Geometry: final body of the model. Coordinates: model frame, mm. A direction names the side the tool comes from. Give positions to 0.01 mm unless a question says otherwise; leave off trailing zeros. Write each loop counter-clockwise with the first axis right and the second up, starting at its lowest first coordinate (ties: lowest second). Pieces come first, ordered by that corner, then holes.
Q1. Section A-A (x = 8.5). Return the cut outline in (y, z).
Q2. Section C-C (y = -94). Return the cut outline in (x, z).
Q3. Mould query, pull axis Y, two halves, no side actions, for faces 3 (the cylindrical face through (8, -89, 22)), 4 (the cylindrical face through (8.28, -82.51, 21.93)), 5 (the flat face through (8, -97.201, 9)), 6 (the flat face through (17, -98, 16)). Classes: +Y half, -Y half, draft (parallel to the pull), parting line (faces both ways), or undercut.
Q4. Section D-D (z = 12). Return the cut outline in (x, y).
Q5. Section B-B (x = 5.5). Return the cut outline in (y, z), plus the area to 3 significant figures.
Q6. Pin query (flat end, axial travel): pin 1 Ø5 at (x, z) = (7.5, 10.5) entering from +Y; pin 2 Ø5 at (x, y) = (7, -83) entering from -Z; pin 3 Ø12 at (y, z) = (-76.5, 18) entering from +X. Return the tip coordinate at first contact, or that it passes through.
Q7. Line query: line 1 (Y direction, x = 8.5, z = 22.15); line 2 (Z direction, x = 8.5, y = -97.6); line 3 (Z direction, x = 5.5, y = -82.5). Output: solid intervals per line, ascending.
Q8. Reachability of faces 1 (the flat face through (8, -86, 22.423)), 2 (the flat face through (8, -85, 21.423)) from +Z, -Z, +X, -X, +Y, -Y: full face, straight path, thin tool, end or side. Return the list, or none.
from build123d import *

# Parameters (mm, degrees)
F1_DEPTH = 17
F2_R     = 1
F3_DEPTH = 1
F4_R     = 1
F5_DEPTH = 1


with BuildPart() as f1:
    # F0 (on Right) → F1 (new body)
    with BuildSketch(Plane.YZ):
        Polygon((-73.201425, 22.422691), (-98.201425, 22.422691), (-98.201425, -2.577309), (-97.201425, -2.577309), (-97.201425, 21.422691), (-73.201425, 21.422691), align=None)
    extrude(amount=F1_DEPTH)

    # F2 (on face) → F3 (cut)
    with BuildSketch(Plane(origin=(0, -97.201425, 0), x_dir=(-1, 0, 0), z_dir=(0, 1, 0))):
        with Locations((-8.5, 5.756025)):
            Circle(F2_R)
        with Locations((-8.5, 14.089358)):
            Circle(F2_R)
    extrude(amount=-F3_DEPTH, mode=Mode.SUBTRACT)

    # F4 (on face) → F5 (cut)
    with BuildSketch(Plane.XY.offset(22.422691)):
        with Locations((8.5, -81.534759)):
            Circle(F4_R)
        with Locations((8.5, -89.868092)):
            Circle(F4_R)
    extrude(amount=-F5_DEPTH, mode=Mode.SUBTRACT)


solid = f1.part
Computed:
1. outline: (-98.2, -2.58) - (-97.2, -2.58) - (-97.2, 4.76) - (-98.2, 4.76) - close; (-98.2, 6.76) - (-97.2, 6.76) - (-97.2, 13.09) - (-98.2, 13.09) - close; (-98.2, 15.09) - (-97.2, 15.09) - (-97.2, 21.42) - (-90.87, 21.42) - (-90.87, 22.42) - (-98.2, 22.42) - close; (-88.87, 21.42) - (-82.53, 21.42) - (-82.53, 22.42) - (-88.87, 22.42) - close; (-80.53, 21.42) - (-73.2, 21.42) - (-73.2, 22.42) - (-80.53, 22.42) - close
2. outline: (0, 21.42) - (17, 21.42) - (17, 22.42) - (0, 22.42) - close
3. face 3: undercut
3. face 4: undercut
3. face 5: +Y half
3. face 6: draft
4. outline: (0, -98.2) - (17, -98.2) - (17, -97.2) - (0, -97.2) - close
5. outline: (-98.2, -2.58) - (-97.2, -2.58) - (-97.2, 21.42) - (-73.2, 21.42) - (-73.2, 22.42) - (-98.2, 22.42) - close
5. area: 49.0 mm2
6. pin 1: stops at y = -97.2
6. pin 2: stops at z = 21.42
6. pin 3: stops at x = 17
7. line 1: y = -98.2 to -90.87, -88.87 to -82.53, -80.53 to -73.2
7. line 2: z = -2.58 to 4.76, 6.76 to 13.09, 15.09 to 22.42
7. line 3: z = 21.42 to 22.42
8. face 1: +Z, +X, -X, +Y, -Y
8. face 2: -Z, +X, -X, +Y
